from build123d import *

# Parameters (mm, degrees)
PAD005_DEPTH           = 6.35
SKETCH004_W            = 12.7
SKETCH004_H            = 6.35
POCKET_DEPTH           = 0.001
POCKET_DEPTH_BACK      = 6.351
LINEARPATTERN_COUNT    = 7
LINEARPATTERN_PITCH    = 25.4
SKETCH005_W            = 6.35
SKETCH005_H            = 12.7
POCKET001_DEPTH        = 0.001
POCKET001_DEPTH_BACK   = 6.351
LINEARPATTERN001_COUNT = 3
LINEARPATTERN001_PITCH = 25.4
POCKET005_DEPTH        = 0.001
POCKET005_DEPTH_BACK   = 6.351


with BuildPart() as part:
    # MirroredSketch001 → Pad005 (new body)
    with BuildSketch(Plane.YZ):
        Polygon((-88.129616, 25.267823), (-25.267823, 88.129616), (-20.777695, 83.639488), (-7.307311, 97.109872), (-11.797439, 101.6), (0, 101.6), (0, 0), (-101.6, 0), (-101.6, 11.797439), (-97.109872, 7.307311), (-83.639488, 20.777695), align=None)
    extrude(amount=PAD005_DEPTH)

    # Sketch004 (on YZ_Plane003 of Origin007) → Pocket (cut, two sides)
    with BuildSketch(Plane.YZ) as pocket_sk:
        with Locations((-6.35, 3.175)):
            Rectangle(SKETCH004_W, SKETCH004_H)
    pocket = extrude(amount=-POCKET_DEPTH, mode=Mode.SUBTRACT) + extrude(pocket_sk.sketch, amount=POCKET_DEPTH_BACK, mode=Mode.SUBTRACT)

    # LinearPattern: Pocket ×7
    with Locations(*[(0, -i * LINEARPATTERN_PITCH, 0) for i in range(1, LINEARPATTERN_COUNT)]):
        add(pocket, mode=Mode.SUBTRACT)

    # Sketch005 (on YZ_Plane003 of Origin007) → Pocket001 (cut, two sides)
    with BuildSketch(Plane.YZ) as pocket001_sk:
        with Locations((-3.175, 25.4)):
            Rectangle(SKETCH005_W, SKETCH005_H)
    pocket001 = extrude(amount=-POCKET001_DEPTH, mode=Mode.SUBTRACT) + extrude(pocket001_sk.sketch, amount=POCKET001_DEPTH_BACK, mode=Mode.SUBTRACT)

    # LinearPattern001: Pocket001 ×3
    with Locations(*[(0, 0, i * LINEARPATTERN001_PITCH) for i in range(1, LINEARPATTERN001_COUNT)]):
        add(pocket001, mode=Mode.SUBTRACT)

    # Sketch012 → Pocket005 (cut, two sides)
    with BuildSketch(Plane.YZ) as pocket005_sk:
        with BuildLine():
            Line((-19.05, 54.519744), (-19.05, 25.4))
            ThreePointArc((-25.4, 19.05), (-20.909872, 20.909872), (-19.05, 25.4))
            Line((-25.4, 19.05), (-54.519744, 19.05))
            ThreePointArc((-59.009872, 29.890128), (-60.386379, 22.96996), (-54.519744, 19.05))
            Line((-59.009872, 29.890128), (-29.890128, 59.009872))
            ThreePointArc((-19.05, 54.519744), (-22.96996, 60.386379), (-29.890128, 59.009872))
        make_face()
    extrude(amount=-POCKET005_DEPTH, mode=Mode.SUBTRACT)
    extrude(pocket005_sk.sketch, amount=POCKET005_DEPTH_BACK, mode=Mode.SUBTRACT)


solid = part.part
Work out the finished part from the listing and answer in its coordinate system (mm). A direction names the side the tool comes from. Round coordinates to 2 decimals unless told otherwise and drop trailing zeros. Write each loop counter-clockwise with the first axis right and the second up, starting at its lowest first coordinate (ties: lowest second). Pieces come first, ordered by that corner, then holes. Notation, with made-up numbers: (46.5, -35.75) -> (70.5, -35.75) arc R27 ccw to (70.5, -16.75) -> close; hole circle Ø1 at (29.5, 48). An arc over 180 degrees is marked (long way). Answer as CSV lines item,"result". Start each with the question number.
(1) The part is cut by section C-C, the plane z = 15.5. Give the vertices of the cut face in (x, y), then the cut area to 3 significant figures.
(2) The part is cut by section B-B, the plane z = 28. Give the vertices of the cut face in (x, y).
(3) Find the intervals of material crossed by probe 1 along Y at (x, z) = (2, 4.5); probe 2 along Z at (x, y) = (2.5, -5.5); probe 3 along Z at (x, y) = (5.75, -34.5), in increasing order.
(4) A tool of negligible diameter and unlimited length cuts with its end or side. For faces 4 (the flat face through (3, -50.8, 3)), 5 (the cylindrical face through (3.13, -20.96, 20.86)), 6 (the flat face through (3, -3, 31.75)), from which of +Z, -Z, +X, -X, +Y, -Y can it reach the whole face along a straight path? Write none if from no direction.
(5) This flat-tipped pin is pushed along its axis until it touches: pin 1 (1.9 mm diameter, centred on x = 3.5, y = -80.5, fed in from -Z). Where does it stop, or does it pass through?
(6) The part is cut by section D-D, the plane y = -15.5. Give the vertices of the cut face in (x, z), then the cut area to 3 significant figures.
(7) The part is cut by section A-A, the plane y = -43. Give the vertices of the cut face in (x, z).
(8) The mould has two halves that part along Z. Classify faces 1 (the flat face through (0, -50, 40)), 2 (the flat face through (3, -70, 0)), 3 (the flat face through (3.1, -44.7, 44.2)): +Z half, -Z half, draft (parallel to the pull), parting line (faces both ways), or undercut.
Output values:
1,outline,"(0, -88.92) -> (6.35, -88.92) -> (6.35, 0) -> (0, 0) -> close"
1,area,"565 mm²"
2,outline,"(0, -85.4) -> (6.35, -85.4) -> (6.35, -60.31) -> (0, -60.31) -> close; (0, -19.05) -> (6.35, -19.05) -> (6.35, -6.35) -> (0, -6.35) -> close"
3,probe 1,"y = -101.6 to -88.9, -76.2 to -63.5, -50.8 to -38.1, -25.4 to -12.7"
3,probe 2,"z = 6.35 to 19.05, 31.75 to 44.45, 57.15 to 69.85, 82.55 to 101.6"
3,probe 3,"z = 6.35 to 19.05, 54.4 to 78.9"
4,face 4,"-Z, +X, -X"
4,face 5,"+X, -X"
4,face 6,"+X, -X, +Y"
5,pin 1,"stops at z = 6.35"
6,outline,"(0, 0) -> (6.35, 0) -> (6.35, 88.92) -> (0, 88.92) -> close"
6,area,"565 mm²"
7,outline,"(0, 0) -> (6.35, 0) -> (6.35, 19.05) -> (0, 19.05) -> close; (0, 45.9) -> (6.35, 45.9) -> (6.35, 70.4) -> (0, 70.4) -> close"
8,face 1,"draft"
8,face 2,"-Z half"
8,face 3,"undercut"
